Autodesk Fusion 360 part; units mm, degrees
sketch "スケッチ1" plane through (0, 0, 0) normal (0, 1, 0) x (1, 0, 0)
  line L0 (0, 0) -> (0, -30)
  line L1 (0, -30) -> (4, -30)
  line L2 (4, -30) -> (4, -4)
  line L3 (4, -27.1719) -> (27.1719, -4)
  line L4 (4, -4) -> (30, -4)
  line L5 (30, -4) -> (30, 0)
  line L6 (30, 0) -> (0, 0)
  dimension "d1" = 30
  dimension "d2" = 30
  dimension "d3" = 4
  dimension "d4" = 4
  dimension "d5" = 32.77
  dimension "d6" = 45
extrude "押し出し1" add sketch "スケッチ1" along normal mid plane 15
extrude "押し出し2" cut sketch "スケッチ1" along normal mid plane 11 contours L2 L3 L4
chamfer "面取り1" distance 6 angle 45 1 edges at (4, 0, 4)
hole "穴1" at (20, 0, 4) direction (0, 0, -1) diameter 5 depth 4 tip angle 118
hole "穴2" at (4, 0, 20) direction (-1, 0, 0) diameter 5 depth 4 tip angle 118
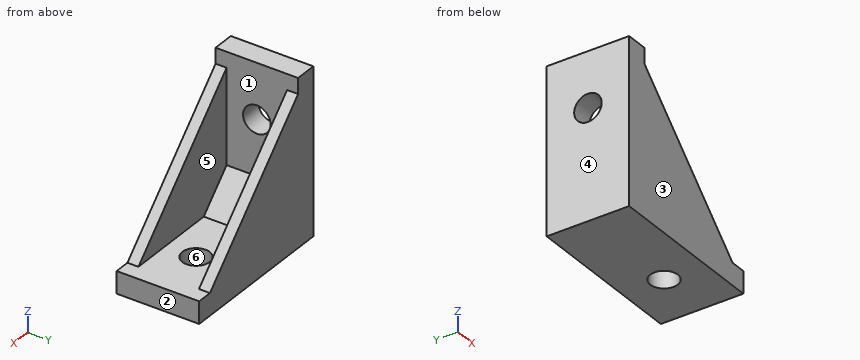
Can you work these out from the model? Positions are in its coordinate system, mm. Face numbers are marked on the shaded views. A direction names the side the tool comes from. Give positions to 0.01 mm unless a question says otherwise; leave off trailing zeros. Loops run counter-clockwise (first coordinate to the right, second up) from the corner with the lowest first, then second, coordinate; pieces in that order, holes last. Notation, with made-up numbers: (-22, -1.75) - (18, -1.75) arc R14 ccw to (18, 3.25) - close; hole circle Ø10 at (-11.75, -11). An arc over 180 degrees is marked (long way). Return JSON: item names as keys, results as strings.
1. I want a section at D-D on z = 3. Please give me the cut outline in (x, y), and give its area (3 significant figures).
Output values:
{"outline": "(0, -7.5) - (30, -7.5) - (30, 7.5) - (0, 7.5) - close; hole circle Ø5 at (20, 0)", "area": "430 mm²"}
2. I want a section at A-A on y = 0. Please give me the cut outline in (x, z), and give its area (3 significant figures).
Output values:
{"outline": "(0, 0) - (17.5, 0) - (17.5, 4) - (10, 4) - (4, 10) - (4, 17.5) - (0, 17.5) - close; (0, 22.5) - (4, 22.5) - (4, 30) - (0, 30) - close; (22.5, 0) - (30, 0) - (30, 4) - (22.5, 4) - close", "area": "202 mm²"}
3. We'd pull the mould along Y, two halves only. Please class the marked faces 3, 4, 5 and 6: +Y half, -Y half, draft (parallel to the pull), parting line (faces both ways), or undercut.
Output values:
{"face 3": "-Y half", "face 4": "draft", "face 5": "undercut", "face 6": "undercut"}
4. If I drill on line 1 (X direction, y = 0, z = 2.65); line 2 (Y direction, x = 3, z = 20), over which ranges is the centre line in solid material (lowest first)?
Output values:
{"line 1": "x = 0 to 17.5, 22.5 to 30", "line 2": "y = -7.5 to -2.5, 2.5 to 7.5"}
5. I want a section at C-C on x = 20. Please give me the cut outline in (y, z).
Output values:
{"outline": "(-7.5, 0) - (-2.5, 0) - (-2.5, 4) - (-5.5, 4) - (-5.5, 11.17) - (-7.5, 11.17) - close; (2.5, 0) - (7.5, 0) - (7.5, 11.17) - (5.5, 11.17) - (5.5, 4) - (2.5, 4) - close"}
6. I want a section at B-B on z = 21.25. Please give me the cut outline in (x, y).
Output values:
{"outline": "(0, -7.5) - (9.92, -7.5) - (9.92, -5.5) - (4, -5.5) - (4, -2.17) - (0, -2.17) - close; (0, 2.17) - (4, 2.17) - (4, 5.5) - (9.92, 5.5) - (9.92, 7.5) - (0, 7.5) - close"}
7. For the marked faces 1 and 2, which set-ups out of +Z, -Z, +X, -X, +Y, -Y let a thin tool reach every point of the face, with its end or its side?
Output values:
{"face 1": "+Z, +X", "face 2": "+Z, -Z, +X, +Y, -Y"}
8. I'm going to push flat-ended pins straight in: pin 1 Ø8 at (x, y) = (20, 0) entering from +Z; pin 2 Ø1 at (x, z) = (25, 7.5) entering from +Y. Where does each tip first touch, or does it pass through?
Output values:
{"pin 1": "stops at z = 4", "pin 2": "passes through"}
